Job drawing, mm, ordinate dimensions from the low corner. One solid piece. Round coordinates to 2 decimals unless told otherwise and drop trailing zeros. Order: outer loops, then holes, each group sorted by start corner. A loop starts at its lowest first (then second) coordinate and runs counter-clockwise, first axis right, second up. Notation, with made-up numbers: (84.5, 87.25) -> (94.5, 87.25) arc R32 cw to (94.5, 118.25) -> close; hole circle Ø2 at (24.5, -37.75). An arc over 180 degrees is marked (long way). Use CSV: the item, a comma, the result in double quotes.
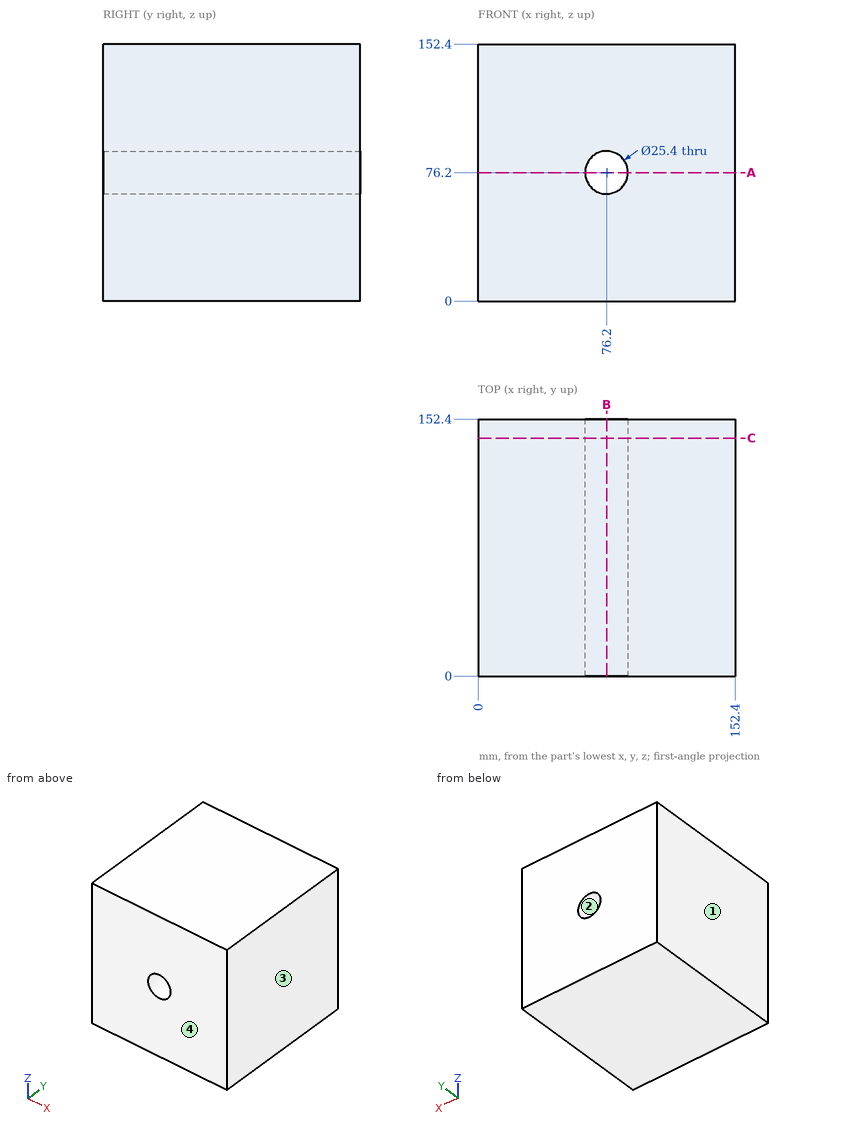
(1) Probe probe 1 along X at (y, z) = (61, 76); probe 2 along Z at (x, y) = (87, 58.5). List the from-to ranges inside material, lowest first. Write a range as [from, to].
Reply:
probe 1,"[0, 63.5], [88.9, 152.4]"
probe 2,"[0, 69.52], [82.88, 152.4]"
(2) Drop a flat-ended pin along its axis: P1, Ø6, axis at x = 103, y = 97.5, coming from the -Z side. Give the stop position or say it passes through.
Reply:
P1,"z = 0"
(3) Cut at C-C, the plane y = 141. Give the cut face in (x, z).
Reply:
outline,"(0, 0) -> (152.4, 0) -> (152.4, 152.4) -> (0, 152.4) -> close; hole circle Ø25.4 at (76.2, 76.2)"
(4) Cut at B-B, the plane x = 76.2. Give the cut face in (y, z).
Reply:
outline,"(0, 0) -> (152.4, 0) -> (152.4, 63.5) -> (0, 63.5) -> close; (0, 88.9) -> (152.4, 88.9) -> (152.4, 152.4) -> (0, 152.4) -> close"
(5) Pull direction X, two halves, no side cores. Call the marked faces 1, 2, 3 and 4: released by +X, released by -X, zero draft, split by the parting line, or undercut.
Reply:
face 1,"released by -X"
face 2,"undercut"
face 3,"released by +X"
face 4,"zero draft"
(6) Cut at A-A, the plane z = 76.2. Give the cut face in (x, y), then the cut area to 3 significant figures.
Reply:
outline,"(0, 0) -> (63.5, 0) -> (63.5, 152.4) -> (0, 152.4) -> close; (88.9, 0) -> (152.4, 0) -> (152.4, 152.4) -> (88.9, 152.4) -> close"
area,"19,400 mm2"
